Can you work these out from the model? Positions are in its coordinate system, mm. Round coordinates to 2 decimals unless told otherwise and drop trailing zeros. Write each loop counter-clockwise with the first axis right and the second up, starting at its lowest first coordinate (ties: lowest second). Pieces come first, ordered by that corner, then holes. Notation, with made-up numbers: M 63.25,-7.5 L 112.25,-7.5 A14 ccw 112.25,15.5 Z; hole C 26,26 d6. An arc over 180 degrees is marked long. Answer as a JSON object with one key per item and string values. Group by question number.
1) Suppose I cut it at B-B, the plane z = 0. Write out the boundary of the cut face in (x, y), and give its area (3 significant figures).
2) Suppose I cut it at C-C, the plane x = 0. Write out the boundary of the cut face in (y, z), and give its area (3 significant figures).
3) Please list where these lines run through material, in increasing order: L1, parallel to Z at x = -13, y = 1.5; L2, parallel to X at y = 0.85, z = -28. Write a range as [from, to].
4) Suppose I cut it at A-A, the plane x = -10. Write out the boundary of the cut face in (y, z), and give its area (3 significant figures).
5) I'm going to push flat-ended pins straight in: pin 1 Ø0.5 at (x, y) = (14, 1) entering from +Z; pin 2 Ø4.5 at (x, z) = (30.445, 0) entering from -Y; pin 3 Ø6.5 at (x, z) = (30.445, 30.445) entering from -Y; pin 4 Ø0.8 at (x, y) = (12, 0.5) entering from -Z. Where does each tip first touch, or does it pass through?
6) Suppose I cut it at D-D, the plane y = 1.3. State how many separate pieces and enclosed holes the cut face has, and give its area (3 significant figures).
from build123d import *

# Parameters (mm, degrees)
SKETCH1_R           = 3.71
SKETCH1_R_2         = 1.925
BOSS_EXTRUDE1_DEPTH = 1.5875
FILLET3_R           = 3
FILLET4_R           = 2


with BuildPart() as part:
    # Sketch1 → Boss-Extrude1 (new body)
    with BuildSketch(Plane(origin=(0, 0, 0), x_dir=(1, 0, 0), z_dir=(0, 1, 0))):
        with BuildLine():
            Line((-25.148871697, 31.27), (-3.478505426, 31.27))
            ThreePointArc((-3.478505426, 31.27), (0, 34.02), (3.478505426, 31.27))
            Line((3.478505426, 31.27), (25.148871697, 31.27))
            ThreePointArc((25.148871697, 31.27), (34.235092347, 34.235092347), (31.27, 25.148871697))
            Line((31.27, 25.148871697), (31.27, 3.478505426))
            ThreePointArc((31.27, 3.478505426), (34.02, 0), (31.27, -3.478505426))
            Line((31.27, -3.478505426), (31.27, -25.148871697))
            ThreePointArc((31.27, -25.148871697), (34.235092347, -34.235092347), (25.148871697, -31.27))
            Line((25.148871697, -31.27), (3.478505426, -31.27))
            ThreePointArc((3.478505426, -31.27), (0, -34.02), (-3.478505426, -31.27))
            Line((-3.478505426, -31.27), (-25.148871697, -31.27))
            ThreePointArc((-25.148871697, -31.27), (-34.235092347, -34.235092347), (-31.27, -25.148871697))
            Line((-31.27, -25.148871697), (-31.27, -3.478505426))
            ThreePointArc((-31.27, -3.478505426), (-34.02, 0), (-31.27, 3.478505426))
            Line((-31.27, 3.478505426), (-31.27, 25.148871697))
            ThreePointArc((-31.27, 25.148871697), (-34.235092347, 34.235092347), (-25.148871697, 31.27))
        make_face()
        with Locations(Location((-30.445, 30.445, 0), (0, 0, 270))):
            Circle(SKETCH1_R, mode=Mode.SUBTRACT)
        with Locations(Location((30.445, 30.445, 0), (0, 0, 90))):
            Circle(SKETCH1_R, mode=Mode.SUBTRACT)
        with Locations(Location((30.445, -30.445, 0), (0, 0, 270))):
            Circle(SKETCH1_R, mode=Mode.SUBTRACT)
        with Locations(Location((-30.445, -30.445, 0), (0, 0, 90))):
            Circle(SKETCH1_R, mode=Mode.SUBTRACT)
        with Locations(Location((0, 30.445, 0), (0, 0, 270))):
            Circle(SKETCH1_R_2, mode=Mode.SUBTRACT)
        with Locations(Location((-30.445, 0, 0), (0, 0, 90))):
            Circle(SKETCH1_R_2, mode=Mode.SUBTRACT)
        with Locations(Location((0, -30.445, 0), (0, 0, 270))):
            Circle(SKETCH1_R_2, mode=Mode.SUBTRACT)
        with Locations(Location((30.445, 0, 0), (0, 0, 90))):
            Circle(SKETCH1_R_2, mode=Mode.SUBTRACT)
        with BuildLine():
            Line((-25.148871697, 29.62), (-3.478505426, 29.62))
            ThreePointArc((-3.478505426, 29.62), (0, 26.87), (3.478505426, 29.62))
            Line((3.478505426, 29.62), (25.148871697, 29.62))
            ThreePointArc((25.148871697, 29.62), (26.654907653, 26.654907653), (29.62, 25.148871697))
            Line((29.62, 25.148871697), (29.62, 3.478505426))
            ThreePointArc((29.62, 3.478505426), (26.87, 0), (29.62, -3.478505426))
            Line((29.62, -3.478505426), (29.62, -25.148871697))
            ThreePointArc((29.62, -25.148871697), (26.654907653, -26.654907653), (25.148871697, -29.62))
            Line((25.148871697, -29.62), (3.478505426, -29.62))
            ThreePointArc((3.478505426, -29.62), (0, -26.87), (-3.478505426, -29.62))
            Line((-3.478505426, -29.62), (-25.148871697, -29.62))
            ThreePointArc((-25.148871697, -29.62), (-26.654907653, -26.654907653), (-29.62, -25.148871697))
            Line((-29.62, -25.148871697), (-29.62, -3.478505426))
            ThreePointArc((-29.62, -3.478505426), (-26.87, 0), (-29.62, 3.478505426))
            Line((-29.62, 3.478505426), (-29.62, 25.148871697))
            ThreePointArc((-29.62, 25.148871697), (-26.654907653, 26.654907653), (-25.148871697, 29.62))
        make_face(mode=Mode.SUBTRACT)
    extrude(amount=BOSS_EXTRUDE1_DEPTH)

    # Fillet3
    fillet3_edges = [part.edges().sort_by_distance(p)[0] for p in [
        (-25.148871697, 0.79375, -31.27),
        (25.148871697, 0.79375, -31.27),
        (31.27, 0.79375, -25.148871697),
        (31.27, 0.79375, 25.148871697),
        (25.148871697, 0.79375, 31.27),
        (-25.148871697, 0.79375, 31.27),
        (-31.27, 0.79375, 25.148871697),
        (-31.27, 0.79375, -25.148871697),
        (-25.148871697, 0.79375, -29.62),
        (-29.62, 0.79375, -25.148871697),
        (-29.62, 0.79375, 25.148871697),
        (-25.148871697, 0.79375, 29.62),
        (25.148871697, 0.79375, 29.62),
        (29.62, 0.79375, 25.148871697),
        (29.62, 0.79375, -25.148871697),
        (25.148871697, 0.79375, -29.62),
    ]]
    fillet(fillet3_edges, radius=FILLET3_R)

    # Fillet4
    fillet4_edges = [part.edges().sort_by_distance(p)[0] for p in [
        (-3.478505426, 0.79375, -31.27),
        (3.478505426, 0.79375, -31.27),
        (31.27, 0.79375, -3.478505426),
        (31.27, 0.79375, 3.478505426),
        (3.478505426, 0.79375, 31.27),
        (-3.478505426, 0.79375, 31.27),
        (-31.27, 0.79375, 3.478505426),
        (-31.27, 0.79375, -3.478505426),
        (-29.62, 0.79375, -3.478505426),
        (-29.62, 0.79375, 3.478505426),
        (-3.478505426, 0.79375, 29.62),
        (3.478505426, 0.79375, 29.62),
        (29.62, 0.79375, 3.478505426),
        (29.62, 0.79375, -3.478505426),
        (3.478505426, 0.79375, -29.62),
        (-3.478505426, 0.79375, -29.62),
    ]]
    fillet(fillet4_edges, radius=FILLET4_R)


solid = part.part
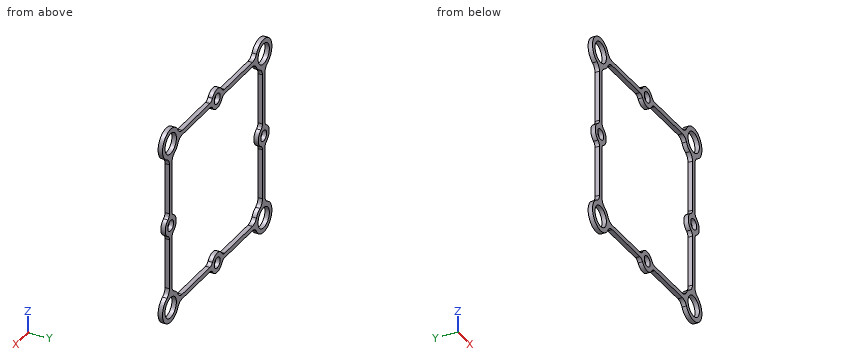
Results:
{
 "1": {"outline": "M -34.02,0 L -32.37,0 L -32.37,1.59 L -34.02,1.59 Z; M -28.52,0 L -26.87,0 L -26.87,1.59 L -28.52,1.59 Z; M 26.87,0 L 28.52,0 L 28.52,1.59 L 26.87,1.59 Z; M 32.37,0 L 34.02,0 L 34.02,1.59 L 32.37,1.59 Z", "area": "10.5 mm^2"},
 "2": {"outline": "M 0,-34.02 L 1.59,-34.02 L 1.59,-32.37 L 0,-32.37 Z; M 0,-28.52 L 1.59,-28.52 L 1.59,-26.87 L 0,-26.87 Z; M 0,26.87 L 1.59,26.87 L 1.59,28.52 L 0,28.52 Z; M 0,32.37 L 1.59,32.37 L 1.59,34.02 L 0,34.02 Z", "area": "10.5 mm^2"},
 "3": {"L1": "[-31.27, -29.62], [29.62, 31.27]", "L2": "[-35.21, -33.24], [-27.65, -25.68], [-2.61, 2.61], [25.68, 27.65], [33.24, 35.21]"},
 "4": {"outline": "M 0,-31.27 L 1.59,-31.27 L 1.59,-29.62 L 0,-29.62 Z; M 0,29.62 L 1.59,29.62 L 1.59,31.27 L 0,31.27 Z", "area": "5.24 mm^2"},
 "5": {"pin 1": "z = 31.27", "pin 2": "y = 0", "pin 3": "through", "pin 4": "z = -31.27"},
 "6": {"separate pieces": "1", "enclosed holes": "9", "area": "603 mm^2"}
}
